Build history of the part. All positions in model axes, mm. Round coordinates to 2 decimals unless told otherwise and drop trailing zeros. Write each loop counter-clockwise with the first axis right and the second up, starting at its lowest first coordinate (ties: lowest second). Pieces come first, ordered by that corner, then holes. Notation, with made-up numbers: (-16.5, 4) -> (42.5, 4) arc R14 ccw to (42.5, 9) -> close; hole circle Ø10 at (5, 83). An arc over 180 degrees is marked (long way). Answer in a Markdown table with one row per item.
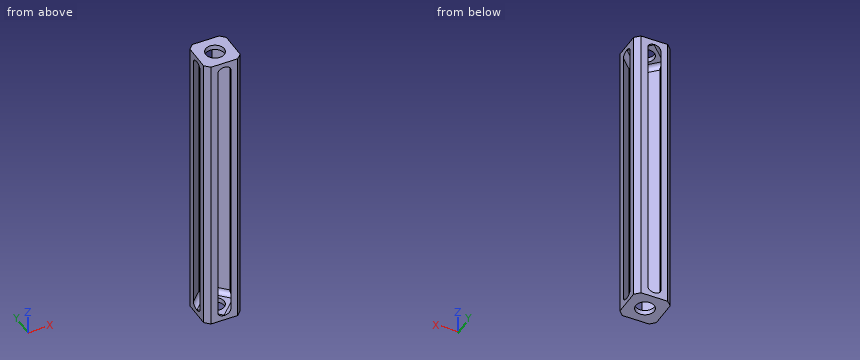
```python
from build123d import *

# Parameters (mm, degrees)
SKETCH1_W           = 19.05
SKETCH1_H           = 19.05
BOSS_EXTRUDE1_DEPTH = 76.2
CHAMFER1_SIZE       = 2.54
SHELL1_T            = -2.54
FILLET1_R           = 2.54
SKETCH3_R           = 4.826
CUT_EXTRUDE1_DEPTH  = 153.9941543


with BuildPart() as part:
    # Sketch1 → Boss-Extrude1 (new, symmetric)
    with BuildSketch(Plane.XY):
        Rectangle(SKETCH1_W, SKETCH1_H)
    extrude(amount=BOSS_EXTRUDE1_DEPTH, both=True)

    # Chamfer1
    chamfer1_edges = [part.edges().sort_by_distance(p)[0] for p in [
        (9.525, -9.525, 0),
        (-9.525, -9.525, 0),
        (-9.525, 9.525, 0),
        (9.525, 9.525, 0),
    ]]
    chamfer(chamfer1_edges, length=CHAMFER1_SIZE)

    # Shell1
    shell1_openings = [part.faces().sort_by_distance(p)[0] for p in [
        (0, -9.525, 0),
        (-9.525, 0, 0),
        (0, 9.525, 0),
        (9.525, 0, 0),
    ]]
    offset(amount=SHELL1_T, openings=shell1_openings, kind=Kind.INTERSECTION)

    # Fillet1
    # the kernel refuses this fillet: 2.54 mm, written as the material it adds along each edge
    with BuildSketch(Plane(origin=(1.097230509, 14.015128061, -73.66), x_dir=(0.7071067811865476, -0.7071067811865476, 0), z_dir=(-0.7071067811865476, -0.7071067811865476, 0))) as fillet1_piece_1_section:
        with BuildLine():
            CenterArc((FILLET1_R, FILLET1_R), FILLET1_R, 180, 90)
            Line((0, FILLET1_R), (0, 0))
            Line((0, 0), (FILLET1_R, 0))
        make_face()
    fillet1_piece_1 = extrude(amount=21.372102448, mode=Mode.PRIVATE)
    fillet1_piece_1 = split(fillet1_piece_1, bisect_by=Plane(origin=(-9.525, 6.009158894, -73.121025702), z_dir=(1, 0, 0)), keep=Keep.TOP, mode=Mode.PRIVATE)
    fillet1_piece_1 = split(fillet1_piece_1, bisect_by=Plane(origin=(-6.009158894, 9.525, -73.121025702), z_dir=(0, -1, 0)), keep=Keep.TOP, mode=Mode.PRIVATE)
    add(fillet1_piece_1)
    with BuildSketch(Plane(origin=(14.015128061, 1.097230509, -73.66), x_dir=(-0.7071067811865476, 0.7071067811865476, 0), z_dir=(-0.7071067811865476, -0.7071067811865476, 0))) as fillet1_piece_2_section:
        with BuildLine():
            CenterArc((FILLET1_R, -FILLET1_R), FILLET1_R, 90, 90)
            Line((0, -FILLET1_R), (0, 0))
            Line((0, 0), (FILLET1_R, 0))
        make_face()
    fillet1_piece_2 = extrude(amount=21.372102448, mode=Mode.PRIVATE)
    fillet1_piece_2 = split(fillet1_piece_2, bisect_by=Plane(origin=(6.009158894, -9.525, -73.121025702), z_dir=(0, 1, 0)), keep=Keep.TOP, mode=Mode.PRIVATE)
    fillet1_piece_2 = split(fillet1_piece_2, bisect_by=Plane(origin=(9.525, -6.009158894, -73.121025702), z_dir=(-1, 0, 0)), keep=Keep.TOP, mode=Mode.PRIVATE)
    add(fillet1_piece_2)
    with BuildSketch(Plane(origin=(14.015128061, -1.097230509, -73.66), x_dir=(-0.7071067811865476, -0.7071067811865476, 0), z_dir=(-0.7071067811865476, 0.7071067811865476, 0))) as fillet1_piece_3_section:
        with BuildLine():
            CenterArc((FILLET1_R, FILLET1_R), FILLET1_R, 180, 90)
            Line((0, FILLET1_R), (0, 0))
            Line((0, 0), (FILLET1_R, 0))
        make_face()
    fillet1_piece_3 = extrude(amount=21.372102448, mode=Mode.PRIVATE)
    fillet1_piece_3 = split(fillet1_piece_3, bisect_by=Plane(origin=(9.525, 6.009158894, -73.121025702), z_dir=(-1, 0, 0)), keep=Keep.TOP, mode=Mode.PRIVATE)
    fillet1_piece_3 = split(fillet1_piece_3, bisect_by=Plane(origin=(6.009158894, 9.525, -73.121025702), z_dir=(0, -1, 0)), keep=Keep.TOP, mode=Mode.PRIVATE)
    add(fillet1_piece_3)
    with BuildSketch(Plane(origin=(1.097230509, -14.015128061, -73.66), x_dir=(0.7071067811865476, 0.7071067811865476, 0), z_dir=(-0.7071067811865476, 0.7071067811865476, 0))) as fillet1_piece_4_section:
        with BuildLine():
            CenterArc((FILLET1_R, -FILLET1_R), FILLET1_R, 90, 90)
            Line((0, -FILLET1_R), (0, 0))
            Line((0, 0), (FILLET1_R, 0))
        make_face()
    fillet1_piece_4 = extrude(amount=21.372102448, mode=Mode.PRIVATE)
    fillet1_piece_4 = split(fillet1_piece_4, bisect_by=Plane(origin=(-9.525, -6.009158894, -73.121025702), z_dir=(1, 0, 0)), keep=Keep.TOP, mode=Mode.PRIVATE)
    fillet1_piece_4 = split(fillet1_piece_4, bisect_by=Plane(origin=(-6.009158894, -9.525, -73.121025702), z_dir=(0, 1, 0)), keep=Keep.TOP, mode=Mode.PRIVATE)
    add(fillet1_piece_4)
    with BuildSketch(Plane(origin=(-14.015128061, -1.097230509, 73.66), x_dir=(0, 0, -1), z_dir=(0.7071067811865476, 0.7071067811865476, 0))) as fillet1_piece_5_section:
        with BuildLine():
            CenterArc((FILLET1_R, -FILLET1_R), FILLET1_R, 90, 90)
            Line((0, -FILLET1_R), (0, 0))
            Line((0, 0), (FILLET1_R, 0))
        make_face()
    fillet1_piece_5 = extrude(amount=21.372102448, mode=Mode.PRIVATE)
    fillet1_piece_5 = split(fillet1_piece_5, bisect_by=Plane(origin=(-9.525, 6.009158894, 73.121025702), z_dir=(1, 0, 0)), keep=Keep.TOP, mode=Mode.PRIVATE)
    fillet1_piece_5 = split(fillet1_piece_5, bisect_by=Plane(origin=(-6.009158894, 9.525, 73.121025702), z_dir=(0, -1, 0)), keep=Keep.TOP, mode=Mode.PRIVATE)
    add(fillet1_piece_5)
    with BuildSketch(Plane(origin=(-1.097230509, 14.015128061, 73.66), x_dir=(0, 0, -1), z_dir=(0.7071067811865476, -0.7071067811865476, 0))) as fillet1_piece_6_section:
        with BuildLine():
            CenterArc((FILLET1_R, -FILLET1_R), FILLET1_R, 90, 90)
            Line((0, -FILLET1_R), (0, 0))
            Line((0, 0), (FILLET1_R, 0))
        make_face()
    fillet1_piece_6 = extrude(amount=21.372102448, mode=Mode.PRIVATE)
    fillet1_piece_6 = split(fillet1_piece_6, bisect_by=Plane(origin=(9.525, 6.009158894, 73.121025702), z_dir=(-1, 0, 0)), keep=Keep.TOP, mode=Mode.PRIVATE)
    fillet1_piece_6 = split(fillet1_piece_6, bisect_by=Plane(origin=(6.009158894, 9.525, 73.121025702), z_dir=(0, -1, 0)), keep=Keep.TOP, mode=Mode.PRIVATE)
    add(fillet1_piece_6)
    with BuildSketch(Plane(origin=(14.015128061, 1.097230509, 73.66), x_dir=(-0.7071067811865476, 0.7071067811865476, 0), z_dir=(-0.7071067811865476, -0.7071067811865476, 0))) as fillet1_piece_7_section:
        with BuildLine():
            CenterArc((FILLET1_R, FILLET1_R), FILLET1_R, 180, 90)
            Line((0, FILLET1_R), (0, 0))
            Line((0, 0), (FILLET1_R, 0))
        make_face()
    fillet1_piece_7 = extrude(amount=21.372102448, mode=Mode.PRIVATE)
    fillet1_piece_7 = split(fillet1_piece_7, bisect_by=Plane(origin=(6.009158894, -9.525, 73.121025702), z_dir=(0, 1, 0)), keep=Keep.TOP, mode=Mode.PRIVATE)
    fillet1_piece_7 = split(fillet1_piece_7, bisect_by=Plane(origin=(9.525, -6.009158894, 73.121025702), z_dir=(-1, 0, 0)), keep=Keep.TOP, mode=Mode.PRIVATE)
    add(fillet1_piece_7)
    with BuildSketch(Plane(origin=(1.097230509, -14.015128061, 73.66), x_dir=(0.7071067811865476, 0.7071067811865476, 0), z_dir=(-0.7071067811865476, 0.7071067811865476, 0))) as fillet1_piece_8_section:
        with BuildLine():
            CenterArc((FILLET1_R, FILLET1_R), FILLET1_R, 180, 90)
            Line((0, FILLET1_R), (0, 0))
            Line((0, 0), (FILLET1_R, 0))
        make_face()
    fillet1_piece_8 = extrude(amount=21.372102448, mode=Mode.PRIVATE)
    fillet1_piece_8 = split(fillet1_piece_8, bisect_by=Plane(origin=(-9.525, -6.009158894, 73.121025702), z_dir=(1, 0, 0)), keep=Keep.TOP, mode=Mode.PRIVATE)
    fillet1_piece_8 = split(fillet1_piece_8, bisect_by=Plane(origin=(-6.009158894, -9.525, 73.121025702), z_dir=(0, 1, 0)), keep=Keep.TOP, mode=Mode.PRIVATE)
    add(fillet1_piece_8)

    # Sketch3 → Cut-Extrude1 (cut, through all)
    with BuildSketch(Plane.XY.offset(76.2)):
        Circle(SKETCH3_R)
    extrude(amount=-CUT_EXTRUDE1_DEPTH, mode=Mode.SUBTRACT)


solid = part.part
```
Q1. Drop a flat-ended pin along its axis: P1, Ø8.5, axis at x = 0, y = 0, coming from the +Z side. Give the stop position or say it passes through.
A:
| item | result |
|---|---|
| P1 | through |
Q2. Saw through at A-A on z = 11.5. Write the cut outline in (x, y) (3 decimals).
A:
| item | result |
|---|---|
| outline | (-9.525, -6.985) -> (-6.985, -9.525) -> (-3.393, -9.525) -> (-9.525, -3.393) -> close; (-9.525, 3.393) -> (-3.393, 9.525) -> (-6.985, 9.525) -> (-9.525, 6.985) -> close; (3.393, -9.525) -> (6.985, -9.525) -> (9.525, -6.985) -> (9.525, -3.393) -> close; (3.393, 9.525) -> (9.525, 3.393) -> (9.525, 6.985) -> (6.985, 9.525) -> close |
Q3. Wall check: line 1 (Z direction, x = 0, y = -7.75); line 2 (Y direction, x = 0, z = 74.8) (3 decimals); line 3 (Z direction, x = -7.75, y = 2). Give the ranges that are in metal, low to high. Write a range as [from, to].
A:
| item | result |
|---|---|
| line 1 | [-76.2, -73.66], [73.66, 76.2] |
| line 2 | [-9.525, -4.826], [4.826, 9.525] |
| line 3 | [-76.2, -73.64], [73.64, 76.2] |
